Autodesk Inventor part; units mm, degrees
ref_plane "YZ Plane" through (0, 0, 0) normal (1, 0, 0) x (0, 1, 0)
ref_plane "XZ Plane" through (0, 0, 0) normal (0, 1, 0) x (-1, 0, 0)
ref_plane "XY Plane" through (0, 0, 0) normal (0, 0, 1) x (1, 0, 0)
sketch "Esboço1" plane through (0, 0, 0) normal (0, 0, 1) x (1, 0, 0)
  line L0 (2.9, 0) -> (65.7, 0)
  line L1 (2.9, 0) -> (2.7, 0)
  line L2 (65.7, 0) -> (65.9, 0)
  line L3 (4.6, 4.8) -> (64, 4.8)
  line L4 (64, 4.8) -> (64.2, 4.8)
  line L5 (65.9, 0) -> (66.1, 0)
  line L6 (66.1, 0) -> (66.1, 2.4)
  line L7 (66.1, 2.4) -> (64.2, 4.3)
  line L8 (64.2, 4.8) -> (64.2, 4.3)
  line L9 (2.9, 0) -> (2.7, 0)
  line L10 (4.6, 4.8) -> (4.4, 4.8)
  line L11 (2.7, 0) -> (2.5, 0)
  line L12 (2.5, 0) -> (2.5, 2.4)
  line L13 (2.5, 2.4) -> (4.4, 4.3)
  line L14 (4.4, 4.8) -> (4.4, 4.3)
  point P0 (61.9143, 91.5369)
extrude "Extrusão1" add sketch "Esboço1" along normal blind 96.6
sketch "Esboço3" plane through (4.4, 4.8, 0) normal (0, 1, 0) x (1, 0, 0)
  line L0 (64.2, -96.6) -> (-4.4, -96.6)
  line L1 (-1.9, -96.6) -> (61.7, -96.6)
  line L2 (29.9, -96.6) -> (29.9, -94.2)
  circle A0 centre (51.4, -94.2) radius 1.45
  line L3 (29.9, -96.6) -> (29.9, -91.8)
  line L4 (29.9, -94.2) -> (51.4, -94.2)
  line L5 (29.9, -94.2) -> (8.4, -94.2)
  circle A1 centre (8.4, -94.2) radius 1.45
  line L6 (0.4, -91.8) -> (59.4, -91.8)
  line L7 (61.7, -96.6) -> (-1.9, -96.6)
  circle A2 centre (29.9, -94.2) radius 1.45
  point P0 (-1.9, 0)
  point P1 (61.7, 0)
  dimension "d104" = 2.4
  dimension "d105" = 2.4
  dimension "d140" = 2.9
extrude "Extrusão3" cut sketch "Esboço3" against normal through all contours A2 L5 L2 | L2 L4 A2 | L5 A2 L3 | L3 A2 L4
sketch "Esboço4" plane through (4.4, 4.8, 0) normal (0, 1, 0) x (1, 0, 0)
  line L0 (-1.9, 0) -> (61.7, 0)
  line L1 (29.9, 0) -> (29.9, -4.8)
  line L2 (29.9, -4.8) -> (29.9, -14.8)
  line L3 (29.9, -14.8) -> (4.9, -14.8)
  line L4 (29.9, -14.8) -> (54.9, -14.8)
  line L5 (4.9, -14.8) -> (4.9, -4.8)
  line L6 (4.9, -4.8) -> (29.9, -4.8)
  line L7 (29.9, -4.8) -> (54.9, -4.8)
  line L8 (54.9, -4.8) -> (54.9, -14.8)
  line L9 (61.7, 0) -> (61.7, -96.6)
  line L10 (61.7, -14.8) -> (-1.9, -14.8)
  line L11 (-1.9, -14.8) -> (-1.9, 0)
  line L12 (-1.9, 0) -> (61.7, 0)
  line L13 (61.7, 0) -> (61.7, -14.8)
  point P0 (-4.4, 0)
  dimension "d51" = 4.8
  dimension "d52" = 10
  dimension "d53" = 25
  dimension "d54" = 25
extrude "Extrusão4" cut sketch "Esboço4" against normal through all
sketch "Esboço5" plane through (4.4, 4.8, 0) normal (0, 1, 0) x (1, 0, 0)
  line L0 (59.8, 0) -> (59.8, -96.6)
  line L1 (0, 0) -> (0, -96.6)
  line L2 (-1.9, -96.6) -> (61.7, -96.6)
  line L3 (-1.9, 0) -> (61.7, 0)
  line L4 (29.9, -85.38) -> (3.23, -85.38)
  line L5 (29.9, -85.38) -> (56.57, -85.38)
  line L6 (3.23, -85.38) -> (3.23, -70.14)
  line L7 (3.23, -70.14) -> (4.23, -70.14)
  line L8 (4.23, -70.14) -> (5.83, -70.14)
  line L9 (56.57, -85.38) -> (56.57, -16.8)
  line L10 (3.23, -70.14) -> (3.23, -16.8)
  line L11 (3.23, -16.8) -> (21.01, -16.8)
  line L12 (3.23, -16.8) -> (48.95, -16.8)
  line L13 (21.01, -16.8) -> (21.01, -17.8)
  line L14 (48.95, -16.8) -> (48.95, -17.8)
  line L15 (21.01, -17.8) -> (21.01, -19.4)
  line L16 (48.95, -17.8) -> (48.95, -19.4)
  circle A0 centre (21.01, -19.4) radius 1.45
  circle A1 centre (48.95, -19.4) radius 1.45
  line L17 (5.83, -70.14) -> (5.83, -70.44)
  circle A2 centre (5.83, -70.44) radius 1.45
  line L18 (53.97, -70.14) -> (53.97, -71.54)
  circle A3 centre (53.97, -71.54) radius 1.45
  line L19 (4.9, -14.8) -> (54.9, -14.8)
  point P0 (-4.4, 0)
  dimension "d60" = 53.34
  dimension "d61" = 15.24
  dimension "d62" = 1
  dimension "d63" = 1.6
  dimension "d64" = 68.58
  dimension "d65" = 17.78
  dimension "d67" = 45.72
  dimension "d69" = 1
  dimension "d70" = 1
  dimension "d71" = 1.6
  dimension "d72" = 1.6
  dimension "d73" = 2.9
  dimension "d74" = 2.9
  dimension "d77" = 68.58
  dimension "d86" = 0.3
  dimension "d87" = 2.9
  dimension "d88" = 1.4
  dimension "d89" = 2.9
extrude "Extrusão5" cut sketch "Esboço5" against normal through all contours A2 | A1 | A0 | A3
sketch "Esboço10" plane through (4.4, 4.8, 96.6) normal (0, 1, 0) x (1, 0, 0)
  circle A0 centre (53.97, 25.06) radius 1.45
  circle A1 centre (5.83, 26.16) radius 1.45
  circle A2 centre (48.95, 77.2) radius 1.45
  line L0 (48.95, 77.2) -> (48.95, 75.75)
  line L1 (48.95, 75.75) -> (48.95, 73.75)
  circle A3 centre (21.01, 77.2) radius 1.45
  line L2 (21.01, 75.75) -> (21.01, 73.75)
  line L3 (59.8, 81.8) -> (59.8, 0)
  line L4 (59.8, 40.9) -> (57.8, 40.9)
  line L5 (0, 81.8) -> (0, 0)
  line L6 (0, 40.9) -> (2, 40.9)
  line L7 (51.4, 3.85) -> (51.4, 5.85)
  line L8 (57.8, 40.9) -> (57.8, 73.75)
  line L9 (57.8, 73.75) -> (48.95, 73.75)
  line L10 (48.95, 73.75) -> (21.01, 73.75)
  line L11 (21.01, 73.75) -> (2, 73.75)
  line L12 (2, 73.75) -> (2, 40.9)
  line L13 (53.97, 28.51) -> (50.52, 28.51)
  line L14 (50.52, 28.51) -> (50.52, 25.06)
  line L15 (51.4, 5.85) -> (57.8, 5.85)
  line L16 (57.8, 40.9) -> (57.8, 28.51)
  line L17 (57.8, 28.51) -> (53.97, 28.51)
  line L18 (57.8, 5.85) -> (57.8, 21.61)
  line L19 (57.8, 21.61) -> (53.97, 21.61)
  line L20 (53.97, 21.61) -> (50.52, 21.61)
  line L21 (50.52, 21.61) -> (50.52, 25.06)
  line L22 (2, 40.9) -> (2, 29.61)
  line L23 (2, 22.71) -> (2, 5.85)
  line L24 (2, 5.85) -> (51.4, 5.85)
  line L25 (2, 29.61) -> (5.83, 29.61)
  line L26 (9.28, 29.61) -> (9.28, 26.16)
  line L27 (9.28, 22.71) -> (5.83, 22.71)
  line L28 (5.83, 22.71) -> (2, 22.71)
  line L29 (9.28, 22.71) -> (9.28, 26.16)
  line L30 (9.28, 29.61) -> (5.83, 29.61)
  line L31 (57.8, 21.61) -> (57.8, 28.51)
  point P0 (-4.4, 96.6)
  dimension "d108" = 2
  dimension "d109" = 2
  dimension "d110" = 2
  dimension "d111" = 2
extrude "Extrusão10" cut sketch "Esboço10" against normal through all contours L9 L8 L16 L17 L13 L14 L21 L20 L19 L18 L15 L24 L23 L28 L27 L29 L26 L30 L25 L22 L12 L11 L10
sketch "Esboço13" plane through (4.4, 4.8, 96.6) normal (0, 1, 0) x (1, 0, 0)
  circle A0 centre (48.95, 77.2) radius 1.45
  line L0 (51.4, 77.2) -> (51.4, 73.75)
  line L1 (51.4, 79.65) -> (51.4, 77.2)
  line L2 (57.8, 77.2) -> (57.8, 79.65)
  line L3 (57.8, 79.65) -> (51.4, 79.65)
  circle A1 centre (21.01, 77.2) radius 1.45
  line L4 (23.46, 77.2) -> (23.46, 73.75)
  line L5 (23.46, 77.2) -> (23.46, 79.65)
  line L6 (46.5, 77.2) -> (46.5, 73.75)
  line L7 (46.5, 77.2) -> (46.5, 79.65)
  line L8 (46.5, 79.65) -> (23.46, 79.65)
  line L9 (17.9739, 79.65) -> (2, 79.65)
  line L10 (2, 73.75) -> (2, 29.61)
  line L11 (2, 79.65) -> (2, 73.75)
  line L12 (2, 73.75) -> (17.9739, 73.75)
  line L13 (18.56, 77.2) -> (18.56, 73.75)
  line L14 (18.56, 73.75) -> (17.9739, 73.75)
  line L15 (18.56, 77.2) -> (18.56, 79.65)
  line L16 (18.56, 79.65) -> (17.9739, 79.65)
  line L17 (9.28, 22.71) -> (9.28, 29.61)
  line L18 (9.28, 29.61) -> (9.28, 28.61)
  line L19 (9.28, 28.61) -> (2, 28.61)
  line L20 (2, 28.61) -> (2, 29.61)
  line L21 (9.28, 29.61) -> (2, 29.61)
  line L22 (57.8, 28.51) -> (57.8, 73.75)
  line L23 (57.8, 77.2) -> (57.8, 73.75)
  line L24 (57.8, 73.75) -> (51.4, 73.75)
  line L25 (2, 73.75) -> (57.8, 73.75)
  line L26 (51.4, 73.75) -> (2, 73.75)
  point P0 (-4.4, 96.6)
  dimension "d139" = 1
extrude "Extrusão12" cut sketch "Esboço13" against normal through all contours L1 L3 L2 L23 L24 L0 | L21 L17 L19 L20 | L14 L12 L11 L9 L16 L15 L13 | L25 L4 L5 L8 L7 L6
sketch "Esboço15" plane through (4.4, 4.8, 96.6) normal (0, 1, 0) x (1, 0, 0)
  circle A0 centre (29.9, 2.4) radius 1.45
  circle A1 centre (29.9, 2.4) radius 1.45
  circle A2 centre (29.9, 2.4) radius 1.95
  point P0 (-4.4, 96.6)
  dimension "d142" = 3.9
extrude "Extrusão13" cut sketch "Esboço15" against normal blind 3
properties part number "tampa"
CAD build for the part. Positions are in the model's coordinates, mm. A direction names the side the tool comes from. Round coordinates to 2 decimals unless told otherwise and drop trailing zeros. Loops run counter-clockwise (first coordinate to the right, second up) from the corner with the lowest first, then second, coordinate; pieces in that order, holes last.
(1) Two-plate mould, pull along Z, no slides. Class faces 1 (the cylindrical face through (9.916, 2.434, 71.856)), 2 (the flat face through (34, 2, 96.6)), 3 (the flat face through (59, 2, 68.09)), 4 (the flat face through (3.4, 3.3, 55.1)): +Z half, -Z half, draft (parallel to the pull), parting line (faces both ways), or undercut.
(2) Cut at C-C (x = 45). Give the cut face in (y, z), plus the area to 3 significant figures.
(3) Cut at A-A (z = 52). Give the cut face in (x, y).
(4) Wall check: line 1 along Z through (x, y) = (34.3, 3.3); line 2 along Z through (x, y) = (55, 0.5); line 3 along X through (y, z) = (1.55, 61). Give the ranges that are in metal, low to high.
(5) Drop flat-ended pins along their axis: pin 1 (1.7 mm diameter, centred on x = 53.35, z = 19.4, fed in from -Y); pin 2 (1.4 mm diameter, centred on y = 3.5, z = 78.5, fed in from +X). Give the stop position or say it passes through.
(6) Which spindle directions (+Z, -Z, +X, -X, +Y, -Y) get a long thin tool onto all of the face, cutting with end or side? Do faces 5 (the flat face through (65.2, 3.3, 55.1)), 6 (the flat face through (54.92, 2, 71)), 7 (the cylindrical face through (36.1, 3.32, 94.95)). Say none if no direction does.
(7) Cut at B-B (y = 0.85). State how many separate pieces and enclosed holes the cut face has, plus the area to 3 significant figures.
(8) Cut at D-D (z = 19.4). Give the cut face in (x, y), plus the area to 3 significant figures.
Findings below:
1. face 1: undercut
1. face 2: +Z half
1. face 3: undercut
1. face 4: draft
2. outline: (0, 14.8) - (4.8, 14.8) - (4.8, 16.95) - (0, 16.95) - close; (0, 90.75) - (4.8, 90.75) - (4.8, 96.6) - (0, 96.6) - close
2. area: 38.4 mm2
3. outline: (2.5, 0) - (6.4, 0) - (6.4, 4.8) - (4.4, 4.8) - (4.4, 4.3) - (2.5, 2.4) - close; (62.2, 0) - (66.1, 0) - (66.1, 2.4) - (64.2, 4.3) - (64.2, 4.8) - (62.2, 4.8) - close
4. line 1: z = 14.8 to 16.95, 90.75 to 92.25, 96.15 to 96.6
4. line 2: z = 14.8 to 22.85, 68.09 to 74.99, 90.75 to 96.6
4. line 3: x = 2.5 to 6.4, 62.2 to 66.1
5. pin 1: passes through
5. pin 2: stops at x = 65.7
6. face 5: +Z, -Z, +X, +Y
6. face 6: +Y, -Y
6. face 7: +Y
7. separate pieces: 1
7. enclosed holes: 6
7. area: 1,200 mm2
8. outline: (2.5, 0) - (6.4, 0) - (6.4, 4.8) - (4.4, 4.8) - (4.4, 4.3) - (2.5, 2.4) - close; (22.96, 0) - (23.96, 0) - (23.96, 4.8) - (22.96, 4.8) - close; (26.86, 0) - (27.86, 0) - (27.86, 4.8) - (26.86, 4.8) - close; (50.9, 0) - (51.9, 0) - (51.9, 4.8) - (50.9, 4.8) - close; (54.8, 0) - (55.8, 0) - (55.8, 4.8) - (54.8, 4.8) - close; (62.2, 0) - (66.1, 0) - (66.1, 2.4) - (64.2, 4.3) - (64.2, 4.8) - (62.2, 4.8) - close
8. area: 51.1 mm2
